Design review of the part shown in the three views and the two pictorial views. Dimensions are in mm from the part's minimum x, y and z. Give positions to 0.01 mm unless a question says otherwise; leave off trailing zeros. Write each loop counter-clockwise with the first axis right and the second up, starting at its lowest first coordinate (ties: lowest second). Pieces come first, ordered by that corner, then holes.
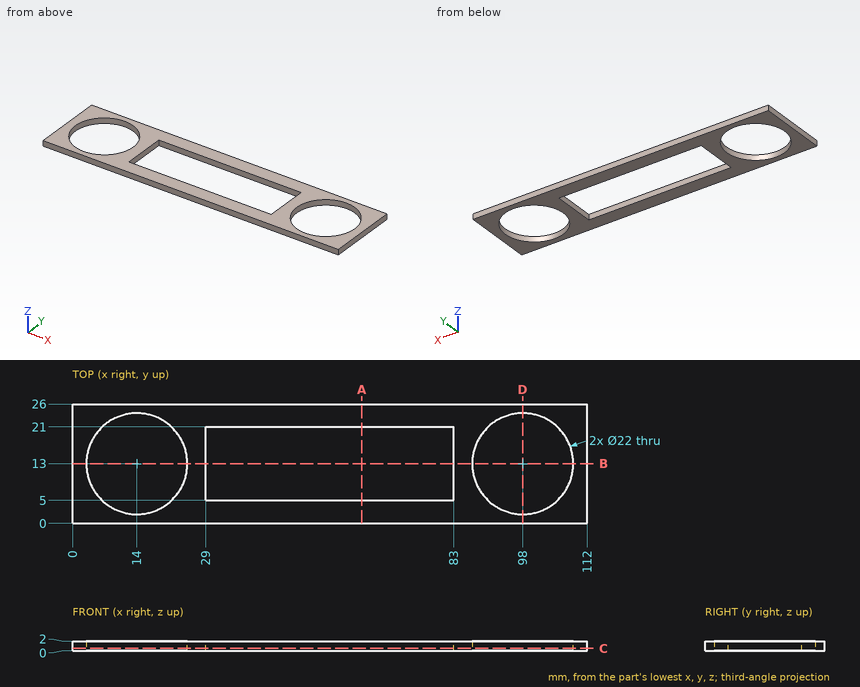
(1) Consider section A-A, the plane x = 63. Give the boundary of the cut face in (y, z).
Resolved:
outline: (0, 0) - (5, 0) - (5, 2) - (0, 2) - close; (21, 0) - (26, 0) - (26, 2) - (21, 2) - close
(2) Consider section D-D, the plane x = 98. Give the boundary of the cut face in (y, z), then the cut area to 3 significant figures.
Resolved:
outline: (0, 0) - (2, 0) - (2, 2) - (0, 2) - close; (24, 0) - (26, 0) - (26, 2) - (24, 2) - close
area: 8.00 mm2
(3) Consider section B-B, the plane y = 13. Give the boundary of the cut face in (x, z).
Resolved:
outline: (0, 0) - (3, 0) - (3, 2) - (0, 2) - close; (25, 0) - (29, 0) - (29, 2) - (25, 2) - close; (83, 0) - (87, 0) - (87, 2) - (83, 2) - close; (109, 0) - (112, 0) - (112, 2) - (109, 2) - close
(4) To check wall thickness, follow L1, parallel to X at y = 12.75, z = 1.55; L2, parallel to Y at x = 35.5, z = 0.5; L3, parallel to X at y = 10, z = 1.55. State the ranges of each line that lie inside material, in increasing order.
Resolved:
L1: x = 0 to 3, 25 to 29, 83 to 87, 109 to 112
L2: y = 0 to 5, 21 to 26
L3: x = 0 to 3.42, 24.58 to 29, 83 to 87.42, 108.58 to 112
(5) Consider section C-C, the plane z = 0.5. Give the boundary of the cut face in (x, y).
Resolved:
outline: (0, 0) - (112, 0) - (112, 26) - (0, 26) - close; hole circle Ø22 at (14, 13); hole (29, 5) - (83, 5) - (83, 21) - (29, 21) - close; hole circle Ø22 at (98, 13)
